```python
from build123d import *

# Parameters (mm, degrees)
SKETCH_1_R          = 12.5
EXTRUDE_1_DEPTH     = 6
CUT_EXTRUDE_1_DEPTH = 3.6
SKETCH_3_R          = 3
CUT_EXTRUDE_2_DEPTH = 2.4


with BuildPart() as part:
    # 草图1 → 凸台-拉伸1 (new body)
    with BuildSketch(Plane.XY):
        Circle(SKETCH_1_R)
    extrude(amount=EXTRUDE_1_DEPTH)

    # 草图2 → 切除-拉伸1 (cut)
    with BuildSketch(Plane.XY.offset(6)):
        Polygon((9.699484522, 0), (4.849742261, 8.4), (-4.849742261, 8.4), (-9.699484522, 0), (-4.849742261, -8.4), (4.849742261, -8.4), align=None)
    extrude(amount=-CUT_EXTRUDE_1_DEPTH, mode=Mode.SUBTRACT)

    # 草图3 → 切除-拉伸2 (cut)
    with BuildSketch(Plane(origin=(0, 0, 0), x_dir=(-1, 0, 0), z_dir=(0, 0, -1))):
        Circle(SKETCH_3_R)
    extrude(amount=-CUT_EXTRUDE_2_DEPTH, mode=Mode.SUBTRACT)


solid = part.part
```
Part model, mm, in its own coordinate system. A direction names the side the tool comes from. Coordinates: 2 decimals unless noted, no trailing zeros. Order: outer loops, then holes, each group sorted by start corner. A loop starts at its lowest first (then second) coordinate and runs counter-clockwise, first axis right, second up. Notation, with made-up numbers: (50.25, 14.25) - (75.25, 14.25) arc R24 ccw to (75.25, 34.25) - close; hole circle Ø6 at (69, 72.5). An arc over 180 degrees is marked (long way). Return JSON: item names as keys, results as strings. Group by question number.
Item 1: Cut at B-B (x = 0). List the corners of the cut face in (y, z), plus the area to 3 significant figures.
Item 2: Cut at C-C (y = -1.5). List the corners of the cut face in (x, z), plus the area to 3 significant figures.
Item 3: Cut at A-A (z = 4.8). List the corners of the cut face in (x, y).
Item 4: Pull direction X, two halves, no side cores. Call faces 1 (the face through (3, -3, 0)), 2 (the face through (11.923, 3.755, 2.958)), 3 (the face through (0, 8.4, 4)): pulls with the +X half, pulls with the -X half, needs draft (parallel to the pull), parting line crosses it, or undercut.
Item 5: Which spindle directions (+Z, -Z, +X, -X, +Y, -Y) get a long thin tool onto all of the face, cutting with end or side? Do faces 4 (the face through (0, 9, 6)), 5 (the face through (-7.31, -4.14, 4.23)). Say none if no direction does.
Item 6: Drill centre lines: probe 1 along Y at (x, z) = (-0.25, 3.6); probe 2 along Y at (x, z) = (0, 0.7); probe 3 along Z at (x, y) = (-7.5, -0.5). Where is each one in solid material? Low to high. Write a range as from..to.
Item 7: Pin check, flat tips, straight feed: pin 1 (1 mm diameter, centred on y = 4.5, z = 2.5, fed in from -X); pin 2 (1.8 mm diameter, centred on x = 2, z = 3.5, fed in from +Y); pin 3 (2 mm diameter, centred on x = -9, z = 0.5, fed in from -Y). Stop position of each tip, or through.
Item 8: Cut at D-D (y = 3.5). List the corners of the cut face in (x, z), plus the area to 3 significant figures.
Check values:
{
 "1": {"outline": "(-12.5, 0) - (-3, 0) - (-3, 2.4) - (-8.4, 2.4) - (-8.4, 6) - (-12.5, 6) - close; (3, 0) - (12.5, 0) - (12.5, 6) - (8.4, 6) - (8.4, 2.4) - (3, 2.4) - close", "area": "75.1 mm2"},
 "2": {"outline": "(-12.41, 0) - (-2.6, 0) - (-2.6, 2.4) - (-8.83, 2.4) - (-8.83, 6) - (-12.41, 6) - close; (2.6, 0) - (12.41, 0) - (12.41, 6) - (8.83, 6) - (8.83, 2.4) - (2.6, 2.4) - close", "area": "72.8 mm2"},
 "3": {"outline": "circle Ø25 at (0, 0); hole (-9.7, 0) - (-4.85, -8.4) - (4.85, -8.4) - (9.7, 0) - (4.85, 8.4) - (-4.85, 8.4) - close"},
 "4": {"face 1": "needs draft", "face 2": "parting line crosses it", "face 3": "undercut"},
 "5": {"face 4": "+Z, +X, -X, +Y, -Y", "face 5": "+Z"},
 "6": {"probe 1": "y = -12.5..-8.4, 8.4..12.5", "probe 2": "y = -12.5..-3, 3..12.5", "probe 3": "z = 0..2.4"},
 "7": {"pin 1": "stops at x = -11.84", "pin 2": "stops at y = 12.45", "pin 3": "stops at y = -9.6"},
 "8": {"outline": "(-12, 0) - (12, 0) - (12, 6) - (7.68, 6) - (7.68, 2.4) - (-7.68, 2.4) - (-7.68, 6) - (-12, 6) - close", "area": "88.7 mm2"}
}
